Design review of the part built by this model. Coordinates are the model's own, in mm. Round coordinates to 2 decimals unless told otherwise and drop trailing zeros. Write each loop counter-clockwise with the first axis right and the second up, starting at its lowest first coordinate (ties: lowest second). Pieces come first, ordered by that corner, then holes. Notation, with made-up numbers: M -18,47.5 L -5,47.5 A31 cw -5,72.5 Z; hole C 41,0 d7. An arc over 180 degrees is marked long. Use CSV: the item, a comma, the result in double quotes.
from build123d import *

# Parameters (mm, degrees)
SKETCH2_W           = 77.47
SKETCH2_H           = 111.76
BOSS_EXTRUDE1_DEPTH = 3.81
SKETCH3_W           = 1.27
SKETCH3_H           = 1.27
BOSS_EXTRUDE2_DEPTH = 111.76
FILLET1_R           = 2.54
CUT_EXTRUDE1_REACH  = 70.829


with BuildPart() as part:
    # Sketch2 → Boss-Extrude1 (new body)
    with BuildSketch(Plane(origin=(0, 0, 0), x_dir=(1, 0, 0), z_dir=(0, 1, 0))):
        Rectangle(SKETCH2_W, SKETCH2_H)
    extrude(amount=BOSS_EXTRUDE1_DEPTH)

    # Sketch3 → Boss-Extrude2 (add)
    with BuildSketch(Plane.XY.offset(55.88)):
        with Locations((-39.37, 0.635)):
            Rectangle(SKETCH3_W, SKETCH3_H)
        with Locations((39.37, 0.635)):
            Rectangle(SKETCH3_W, SKETCH3_H)
    extrude(amount=-BOSS_EXTRUDE2_DEPTH)

    # Fillet1
    fillet1_edges = [part.edges().sort_by_distance(p)[0] for p in [
        (0, 3.81, -55.88),
    ]]
    fillet(fillet1_edges, radius=FILLET1_R)

    # Sketch5 → Cut-Extrude1 (cut, up to next)
    with BuildSketch(Plane(origin=(0, 3.81, 0), x_dir=(1, 0, 0), z_dir=(0, 1, 0)), mode=Mode.PRIVATE) as cut_extrude1_sk1:
        with BuildLine():
            Line((40.005, 55.539704526), (40.005, 55.88))
            Line((40.005, 55.88), (38.735, 55.88))
            ThreePointArc((38.735, 55.88), (39.392400375, 55.793451599), (40.005, 55.539704526))
        make_face()
    cut_extrude1_tool1 = extrude(cut_extrude1_sk1.sketch, amount=-CUT_EXTRUDE1_REACH, mode=Mode.PRIVATE) & part.part
    # Sketch5 → Cut-Extrude1 (cut, up to next)
    with BuildSketch(Plane(origin=(0, 3.81, 0), x_dir=(1, 0, 0), z_dir=(0, 1, 0)), mode=Mode.PRIVATE) as cut_extrude1_sk2:
        with BuildLine():
            ThreePointArc((-40.005, 55.539704526), (-39.392400375, 55.793451599), (-38.735, 55.88))
            Line((-38.735, 55.88), (-40.005, 55.88))
            Line((-40.005, 55.88), (-40.005, 55.539704526))
        make_face()
    cut_extrude1_tool2 = extrude(cut_extrude1_sk2.sketch, amount=-CUT_EXTRUDE1_REACH, mode=Mode.PRIVATE) & part.part
    add(cut_extrude1_tool1.solids().sort_by_distance((39.69191, 3.81, -55.779201))[0], mode=Mode.SUBTRACT)
    add(cut_extrude1_tool2.solids().sort_by_distance((-39.69191, 3.81, -55.779201))[0], mode=Mode.SUBTRACT)


solid = part.part
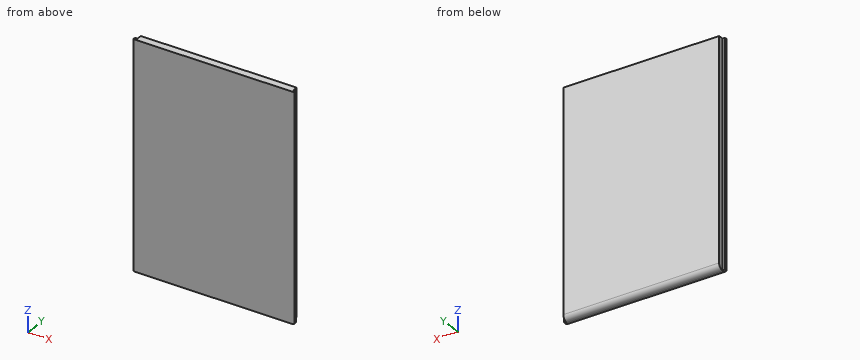
1) Add section B-B on y = 2.25. Write out the cut boundary in (x, z) (3 decimals), then the cut area to 3 significant figures.
Answers:
outline,"M -38.735,-55.683 L 38.735,-55.683 L 38.735,55.88 L -38.735,55.88 Z"
area,"8,640 mm²"
2) For pin 1 Ø1.3 at (y, z) = (3, -15) entering from +X (3 decimals); pin 2 Ø2 at (y, z) = (3.5, 25.5) entering from -X (3 decimals); pin 3 Ø1.4 at (x, z) = (-39.5, -24.5) entering from +Y, all flat-tipped, find the tip position at first contact; note any pin that passes through.
Answers:
pin 1,"x = 38.735"
pin 2,"x = -38.735"
pin 3,"y = 1.27"
3) Wall thickness on line 1 along Z through (x, y) = (28, 1.55); line 2 along X through (y, z) = (1.35, -4.5) (3 decimals); line 3 along Z through (x, y) = (-10, 3.3): over which ranges is each line inside the solid? List them lowest first. Write a range as [from, to].
Answers:
line 1,"[-55.86, 55.88]"
line 2,"[-38.735, 38.735]"
line 3,"[-54.87, 55.88]"
4) Add section A-A on z = -26. Write out the cut boundary in (x, y) (3 decimals).
Answers:
outline,"M -40.005,0 L 40.005,0 L 40.005,1.27 L 38.735,1.27 L 38.735,3.81 L -38.735,3.81 L -38.735,1.27 L -40.005,1.27 Z"
